from build123d import *

# Parameters (mm, degrees)
F1_DEPTH = 50.8
F3_DEPTH = 50.801


with BuildPart() as f1:
    # F0 (on Top) → F1 (new body)
    with BuildSketch(Plane.XY):
        Polygon((-20.32, -25.4), (17.78, -25.4), (17.78, -12.7), (0, -12.7), (0, 12.7), (17.78, 12.7), (17.78, 25.4), (-20.32, 25.4), (-20.32, 12.7), (-33.02, 12.7), (-33.02, 0), (-33.02, -12.7), (-20.32, -12.7), align=None)
    extrude(amount=F1_DEPTH)

    # F2 (on face) → F3 (cut, through all)
    with BuildSketch(Plane.XZ.offset(25.4)):
        Polygon((17.78, 50.8), (-7.62, 50.8), (17.78, 25.4), align=None)
    extrude(amount=-F3_DEPTH, mode=Mode.SUBTRACT)


solid = f1.part
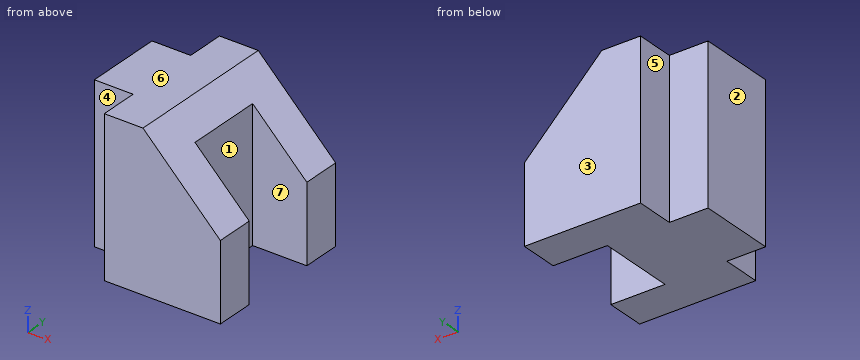
Verification items for the finished model (mm, model axes). Face numbers are marked on the shaded views. A direction names the side the tool comes from. Give positions to 0.01 mm unless a question says otherwise; leave off trailing zeros. Write each loop counter-clockwise with the first axis right and the second up, starting at its lowest first coordinate (ties: lowest second). Pieces come first, ordered by that corner, then holes. Notation, with made-up numbers: M -33,82 L -12,82 A5 ccw -12,91 Z; hole C -29.5,-18.5 d1. An arc over 180 degrees is marked long. Use CSV: the item, a comma, the result in double quotes.
1) Cross-section at A-A (x = 5.5). Enter the section's corners in (y, z), plus the area to 3 significant figures.
Final values:
outline,"M -25.4,0 L -12.7,0 L -12.7,37.68 L -25.4,37.68 Z; M 12.7,0 L 25.4,0 L 25.4,37.68 L 12.7,37.68 Z"
area,"957 mm²"
2) Material ranges on line 1 along Y through (x, z) = (9, 6); line 2 along X through (y, z) = (15.5, 3.5); line 3 along X through (y, z) = (11, 16), recorded low to high.
Final values:
line 1,"-25.4 to -12.7, 12.7 to 25.4"
line 2,"-20.32 to 17.78"
line 3,"-33.02 to 0"
3) Release check for a two-part mould opening along Y. For the marked faces 1, 2 and 3 record: released by +Y, released by -Y, zero draft, split by the parting line, or undercut.
Final values:
face 1,"undercut"
face 2,"zero draft"
face 3,"released by +Y"
4) Cross-section at C-C (y = -1.5). Enter the section's corners in (x, z).
Final values:
outline,"M -33.02,0 L 0,0 L 0,43.18 L -7.62,50.8 L -33.02,50.8 Z"
5) Access from +Z, -Z, +X, -X, +Y, -Y to the whole of each face (thin tool, end or side, straight path). Record for the marked faces 4, 5, 6 and 7.
Final values:
face 4,"+Z, -Z, -X, -Y"
face 5,"+Z, -Z, -X, +Y"
face 6,"+Z, +X, -X, +Y, -Y"
face 7,"+Z, -Z, +X"
6) Cross-section at D-D (x = 11.5). Enter the section's corners in (y, z).
Final values:
outline,"M -25.4,0 L -12.7,0 L -12.7,31.68 L -25.4,31.68 Z; M 12.7,0 L 25.4,0 L 25.4,31.68 L 12.7,31.68 Z"
7) Go/stop test with flat-tipped pins: pin 1 Ø3 at (y, z) = (12.5, 27.5) entering from +X; pin 2 Ø10 at (x, z) = (-29, 13) entering from +Y; pin 3 Ø10 at (y, z) = (20, 18.5) entering from -X. Record where each tip stops, or that it passes through.
Final values:
pin 1,"x = 17.17"
pin 2,"y = 12.7"
pin 3,"x = -20.32"
8) Cross-section at B-B (z = 37.5). Enter the section's corners in (x, y), plus the area to 3 significant figures.
Final values:
outline,"M -33.02,-12.7 L -20.32,-12.7 L -20.32,-25.4 L 5.68,-25.4 L 5.68,-12.7 L 0,-12.7 L 0,12.7 L 5.68,12.7 L 5.68,25.4 L -20.32,25.4 L -20.32,12.7 L -33.02,12.7 Z"
area,"1,500 mm²"
